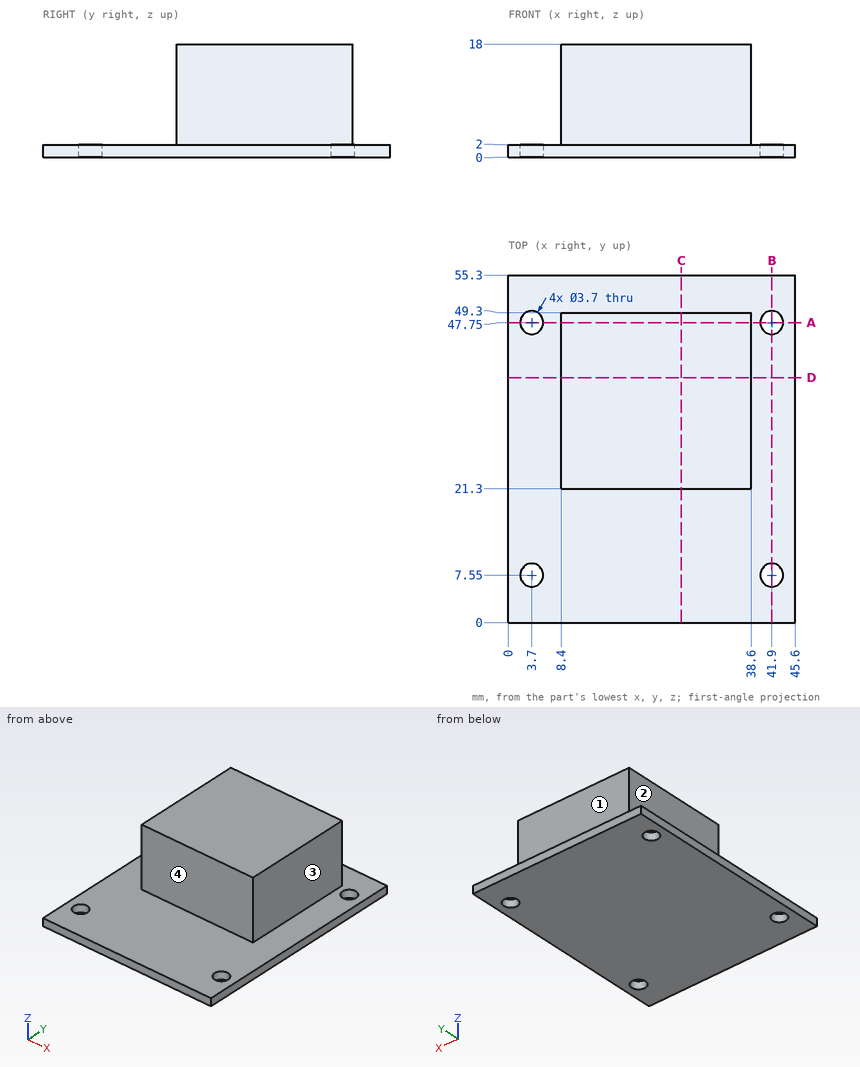
Geometry check sheet. Reference: drawing and pictorial views, mm from the part's lowest x, y, z. A direction names the side the tool comes from. Round coordinates to 2 decimals unless told otherwise and drop trailing zeros. Loops run counter-clockwise (first coordinate to the right, second up) from the corner with the lowest first, then second, coordinate; pieces in that order, holes last. Notation, with made-up numbers: (29, 14.25) - (66, 14.25) arc R18 ccw to (66, 45.25) - close; hole circle Ø1 at (57, 51). An arc over 180 degrees is marked (long way). Answer as CSV lines item,"result".
(1) Cross-section at D-D, the plane y = 39. Enter the section's corners in (x, z), and give its area (3 significant figures).
Output values:
outline,"(0, 0) - (45.6, 0) - (45.6, 2) - (38.6, 2) - (38.6, 18) - (8.4, 18) - (8.4, 2) - (0, 2) - close"
area,"574 mm²"
(2) Cross-section at A-A, the plane y = 47.75. Enter the section's corners in (x, z), and give its area (3 significant figures).
Output values:
outline,"(0, 0) - (1.85, 0) - (1.85, 2) - (0, 2) - close; (5.55, 0) - (40.05, 0) - (40.05, 2) - (38.6, 2) - (38.6, 18) - (8.4, 18) - (8.4, 2) - (5.55, 2) - close; (43.75, 0) - (45.6, 0) - (45.6, 2) - (43.75, 2) - close"
area,"560 mm²"
(3) Cross-section at B-B, the plane x = 41.9. Enter the section's corners in (y, z), and give its area (3 significant figures).
Output values:
outline,"(0, 0) - (5.7, 0) - (5.7, 2) - (0, 2) - close; (9.4, 0) - (45.9, 0) - (45.9, 2) - (9.4, 2) - close; (49.6, 0) - (55.3, 0) - (55.3, 2) - (49.6, 2) - close"
area,"95.8 mm²"
(4) Material ranges on line 1 along Y through (x, z) = (3.7, 0.7); line 2 along Z through (x, y) = (18.5, 10.5); line 3 along Y through (x, z) = (24.5, 6.5), recorded low to high.
Output values:
line 1,"y = 0 to 5.7, 9.4 to 45.9, 49.6 to 55.3"
line 2,"z = 0 to 2"
line 3,"y = 21.3 to 49.3"
(5) Cross-section at C-C, the plane x = 27.5. Enter the section's corners in (y, z), and give its area (3 significant figures).
Output values:
outline,"(0, 0) - (55.3, 0) - (55.3, 2) - (49.3, 2) - (49.3, 18) - (21.3, 18) - (21.3, 2) - (0, 2) - close"
area,"559 mm²"
(6) Depth check by flat-ended pin: pin 1 Ø4 at (x, z) = (27, 9.5) entering from -Y; pin 2 Ø1.5 at (x, y) = (14.5, 23.5) entering from -Z; pin 3 Ø5 at (x, z) = (24, 9) entering from +Y; pin 4 Ø6 at (x, y) = (3.7, 7.55) entering from +Z. Enter the tip coordinate at first touch or a pass-through.
Output values:
pin 1,"stops at y = 21.3"
pin 2,"stops at z = 0"
pin 3,"stops at y = 49.3"
pin 4,"stops at z = 2"
(7) Set-up check for the marked faces 1, 2, 3 and 4: record each of +Z, -Z, +X, -X, +Y, -Y from which the full face is reachable in a straight line by a thin tool's end or side.
Output values:
face 1,"+Z, +X, -X, +Y"
face 2,"+Z, -X, +Y, -Y"
face 3,"+Z, +X, +Y, -Y"
face 4,"+Z, +X, -X, -Y"
